The listing builds one solid part. Answer for the finished solid, in the listing's coordinates (mm). A direction names the side the tool comes from. Give positions to 0.01 mm unless a question says otherwise; leave off trailing zeros. Order: outer loops, then holes, each group sorted by start corner. A loop starts at its lowest first (then second) coordinate and runs counter-clockwise, first axis right, second up. Notation, with made-up numbers: (-36, 6.5) - (4, 6.5) arc R12 cw to (4, 21.5) - close; hole circle Ø6 at (-4.5, 46.25). An arc over 180 degrees is marked (long way). Use a Markdown table: item, result. Add a question column.
1) Flat-ended cylindrical pins translate along their axes: pin 1 (3 mm diameter, centred on y = -9.35, z = 0, fed in from -X); pin 2 (8 mm diameter, centred on x = 11, z = -2.5, fed in from +Y); pin 3 (3 mm diameter, centred on x = -1, z = -3.5, fed in from -Y); pin 4 (8 mm diameter, centred on x = 16, y = -2.5, fed in from -Z). Find the tip coordinate at first contact, or state that the pin passes through.
2) The mould has two halves that part along Y. Classify faces 1 (the face through (29.06, -27.47, -2.57)), 2 (the face through (-5, 0, -2.45)), 3 (the face through (-4.7, 3.74, -0.93)): released by +Y, released by -Y, zero draft, split by the parting line, or undercut.
3) Straight lines are drawn through the part: line 1 (Y direction, x = 23.75, z = 0); line 2 (Y direction, x = 27.7, z = 0); line 3 (X direction, y = -14, z = 7.25). For each, find the intervals that lie inside material, in ascending order.
4) Find section D-D, the plane y = 7. Determine the outline of the cut face in (x, z), plus the area to 3 significant figures.
5) For faces 4 (the face through (-9, -5, 0)), 5 (the face through (-4.7, -3.742, 2.473)), 6 (the face through (10, -4.95, 0)), 7 (the face through (29.06, -27.47, 2.57)), determine the directions among +Z, -Z, +X, -X, +Y, -Y from which every point of the face is accessible in a straight line to the end or side of a thin tool.
6) Find section A-A, the plane y = -20.6. Determine the outline of the cut face in (x, z), plus the area to 3 significant figures.
7) Find section C-C, the plane y = -9.35. Determine the outline of the cut face in (x, z).
from build123d import *

# Parameters (mm, degrees)
SKETCH1_W            = 20
SKETCH1_H            = 20
BOSS_EXTRUDE1_DEPTH  = 20
SKETCH2_W            = 45
SKETCH2_H            = 70
BOSS_EXTRUDE2_DEPTH  = 12
CUT_EXTRUDE1_DEPTH   = 5.8
FILLET1_R            = 3.6
FILLET2_R            = 10
SKETCH5_R            = 3.9
CUT_EXTRUDE2_DEPTH   = 53.490475326
CUT_EXTRUDE3_REACH   = 51.17
SKETCH6_R            = 1.75
SKETCH7_W            = 12
SKETCH7_H            = 45
CUT_EXTRUDE4_DEPTH   = 4.8
SKETCH9_W            = 12
SKETCH9_H            = 45
CUT_EXTRUDE5_DEPTH   = 23.8
SKETCH10_W           = 12.5
SKETCH10_H           = 41.4
CUT_EXTRUDE6_DEPTH   = 23.8
SKETCH11_W           = 20
SKETCH11_H           = 1.2
CUT_EXTRUDE7_DEPTH   = 23.8
BOSS_EXTRUDE3_START  = 20
SKETCH12_W           = 20
SKETCH12_H           = 20
SKETCH12_R           = 3.9
BOSS_EXTRUDE3_DEPTH  = 20
SKETCH13_W           = 20.2
SKETCH13_H           = 20.2
SKETCH13_R           = 3.9
BOSS_EXTRUDE4_DEPTH  = 40
SKETCH14_W           = 12
SKETCH14_H           = 20
BOSS_EXTRUDE5_DEPTH  = 0.1
SKETCH17_R           = 4.83091966
BOSS_EXTRUDE8_DEPTH  = 39
SKETCH18_W           = 25.638800628
SKETCH18_H           = 46.621959296
CUT_EXTRUDE8_DEPTH   = 43
SKETCH19_W           = 9.9
SKETCH19_H           = 9.9
BOSS_EXTRUDE9_DEPTH  = 26.27
BOSS_EXTRUDE10_DEPTH = 2.9
SKETCH21_W           = 10
SKETCH21_H           = 10
BOSS_EXTRUDE11_DEPTH = 5


with BuildPart() as part:
    # Sketch1 → Boss-Extrude1 (new body)
    with BuildSketch(Plane(origin=(0, 0, 0), x_dir=(0, 0, -1), z_dir=(1, 0, 0))):
        Rectangle(SKETCH1_W, SKETCH1_H)
    extrude(amount=BOSS_EXTRUDE1_DEPTH)

    # Sketch2 → Boss-Extrude2 (add)
    with BuildSketch(Plane(origin=(20, 0, 0), x_dir=(0, 0, -1), z_dir=(1, 0, 0))):
        Rectangle(SKETCH2_W, SKETCH2_H)
    extrude(amount=BOSS_EXTRUDE2_DEPTH)

    # Sketch4 → Cut-Extrude1 (cut)
    with BuildSketch(Plane(origin=(32, 0, 0), x_dir=(0, 0, -1), z_dir=(1, 0, 0))):
        with BuildLine():
            Line((3.6, -28.55), (-3.6, -28.55))
            Line((-3.6, -28.55), (-3.6, -7.311805523))
            ThreePointArc((-3.6, -7.311805523), (0, 8.15), (3.6, -7.311805523))
            Line((3.6, -7.311805523), (3.6, -28.55))
        make_face()
    extrude(amount=-CUT_EXTRUDE1_DEPTH, mode=Mode.SUBTRACT)

    # Fillet1
    fillet1_edges = [part.edges().sort_by_distance(p)[0] for p in [
        (29.1, -28.55, 3.6),
        (29.1, -28.55, -3.6),
    ]]
    fillet(fillet1_edges, radius=FILLET1_R - 0.0001)  # a hair under: the kernel refuses the full size

    # Fillet2
    fillet2_edges = [part.edges().sort_by_distance(p)[0] for p in [
        (29.1, -7.311805523, 3.6),
        (29.1, -7.311805523, -3.6),
    ]]
    fillet(fillet2_edges, radius=FILLET2_R)

    # Sketch5 → Cut-Extrude2 (cut, through all)
    with BuildSketch(Plane.ZY):
        Circle(SKETCH5_R)
    extrude(amount=-CUT_EXTRUDE2_DEPTH, mode=Mode.SUBTRACT)

    # Sketch6 → Cut-Extrude3 (cut, up to next)
    with BuildSketch(Plane(origin=(26.2, 0, 0), x_dir=(0, 0, -1), z_dir=(1, 0, 0)), mode=Mode.PRIVATE) as cut_extrude3_sk1:
        with Locations((0, -20.6)):
            Circle(SKETCH6_R)
    cut_extrude3_tool1 = extrude(cut_extrude3_sk1.sketch, amount=-CUT_EXTRUDE3_REACH, mode=Mode.PRIVATE) & part.part
    # Sketch6 → Cut-Extrude3 (cut, up to next)
    with BuildSketch(Plane(origin=(26.2, 0, 0), x_dir=(0, 0, -1), z_dir=(1, 0, 0)), mode=Mode.PRIVATE) as cut_extrude3_sk2:
        with Locations((0, -9.35)):
            Circle(SKETCH6_R)
    cut_extrude3_tool2 = extrude(cut_extrude3_sk2.sketch, amount=-CUT_EXTRUDE3_REACH, mode=Mode.PRIVATE) & part.part
    add(cut_extrude3_tool1.solids().sort_by_distance((26.2, -20.6, 0))[0], mode=Mode.SUBTRACT)
    add(cut_extrude3_tool2.solids().sort_by_distance((26.2, -9.35, 0))[0], mode=Mode.SUBTRACT)

    # Sketch7 → Cut-Extrude4 (cut)
    with BuildSketch(Plane.XZ.offset(35)):
        with Locations((26, 0)):
            Rectangle(SKETCH7_W, SKETCH7_H)
    extrude(amount=-CUT_EXTRUDE4_DEPTH, mode=Mode.SUBTRACT)

    # Sketch9 → Cut-Extrude5 (cut)
    with BuildSketch(Plane(origin=(0, 35, 0), x_dir=(1, 0, 0), z_dir=(0, 1, 0))):
        with Locations((26, 0)):
            Rectangle(SKETCH9_W, SKETCH9_H)
    extrude(amount=-CUT_EXTRUDE5_DEPTH, mode=Mode.SUBTRACT)

    # Sketch10 → Cut-Extrude6 (cut)
    with BuildSketch(Plane.ZY.offset(-20)):
        with Locations((-16.25, -9.5)):
            Rectangle(SKETCH10_W, SKETCH10_H)
        with Locations((16.25, -9.5)):
            Rectangle(SKETCH10_W, SKETCH10_H)
    extrude(amount=-CUT_EXTRUDE6_DEPTH, mode=Mode.SUBTRACT)

    # Sketch11 → Cut-Extrude7 (cut)
    with BuildSketch(Plane.ZY.offset(-20)):
        with Locations((0, 10.6)):
            Rectangle(SKETCH11_W, SKETCH11_H)
    extrude(amount=-CUT_EXTRUDE7_DEPTH, mode=Mode.SUBTRACT)

    # Sketch12 → Boss-Extrude3 (add)
    with BuildSketch(Plane.ZY.offset(BOSS_EXTRUDE3_START)):
        Rectangle(SKETCH12_W, SKETCH12_H)
        Circle(SKETCH12_R, mode=Mode.SUBTRACT)
    extrude(amount=-BOSS_EXTRUDE3_DEPTH)

    # Sketch13 → Boss-Extrude4 (add)
    with BuildSketch(Plane.ZY.offset(20)):
        Rectangle(SKETCH13_W, SKETCH13_H)
        Circle(SKETCH13_R, mode=Mode.SUBTRACT)
    extrude(amount=-BOSS_EXTRUDE4_DEPTH)

    # Sketch14 → Boss-Extrude5 (add)
    with BuildSketch(Plane(origin=(0, 10, 0), x_dir=(1, 0, 0), z_dir=(0, 1, 0))):
        with Locations((26, 0)):
            Rectangle(SKETCH14_W, SKETCH14_H)
    extrude(amount=BOSS_EXTRUDE5_DEPTH)

    # Sketch17 → Boss-Extrude8 (add)
    with BuildSketch(Plane.ZY.offset(20)):
        Circle(SKETCH17_R)
    extrude(amount=-BOSS_EXTRUDE8_DEPTH)

    # Sketch18 → Cut-Extrude8 (cut)
    with BuildSketch(Plane.ZY.offset(20)):
        with Locations((-2.719400314, -13.210979648)):
            Rectangle(SKETCH18_W, SKETCH18_H)
    extrude(amount=-CUT_EXTRUDE8_DEPTH, mode=Mode.SUBTRACT)

    # Sketch19 → Boss-Extrude9 (add)
    with BuildSketch(Plane.ZY.offset(-23)):
        Rectangle(SKETCH19_W, SKETCH19_H)
    extrude(amount=BOSS_EXTRUDE9_DEPTH)

    # Sketch20 → Boss-Extrude10 (add)
    with BuildSketch(Plane.ZY.offset(3.27)):
        Polygon((0.55, 4.95), (-2.45, 2.5), (-2.45, -2.5), (0.55, -4.95), (4.45, -2.5), (4.45, 2.5), align=None)
    extrude(amount=BOSS_EXTRUDE10_DEPTH)

    # Sketch21 → Boss-Extrude11 (add)
    with BuildSketch(Plane.ZY.offset(6.17)):
        Rectangle(SKETCH21_W, SKETCH21_H)
    extrude(amount=BOSS_EXTRUDE11_DEPTH)


solid = part.part
The answers:
| question | item | result |
|---|---|---|
| 1 | pin 1 | through |
| 1 | pin 2 | y = 4.95 |
| 1 | pin 3 | y = -4.95 |
| 1 | pin 4 | z = -4.95 |
| 2 | face 1 | undercut |
| 2 | face 2 | zero draft |
| 2 | face 3 | released by +Y |
| 3 | line 1 | -30.2 to -22.35, -18.85 to -11.1, -7.6 to -3.9, 3.9 to 10.1 |
| 3 | line 2 | -30.2 to -28.55, 8.15 to 10.1 |
| 3 | line 3 | 23 to 32 |
| 4 | outline | (23, -10) - (32, -10) - (32, -4.17) - (26.2, -4.17) - (26.2, 4.17) - (32, 4.17) - (32, 10) - (23, 10) - close |
| 4 | area | 132 mm2 |
| 5 | face 4 | +Z, -Z, -X, -Y |
| 5 | face 5 | +Z, -Y |
| 5 | face 6 | +Z, -Z, -Y |
| 5 | face 7 | +X |
| 6 | outline | (23, -10) - (32, -10) - (32, -3.6) - (26.2, -3.6) - (26.2, -1.75) - (23, -1.75) - close; (23, 1.75) - (26.2, 1.75) - (26.2, 3.6) - (32, 3.6) - (32, 10) - (23, 10) - close |
| 6 | area | 127 mm2 |
| 7 | outline | (23, -10) - (32, -10) - (32, -3.96) - (26.2, -3.96) - (26.2, -1.75) - (23, -1.75) - close; (23, 1.75) - (26.2, 1.75) - (26.2, 3.96) - (32, 3.96) - (32, 10) - (23, 10) - close |
